Geometry check sheet. Reference: the model listing, model coordinates, mm. Face numbers are marked on the shaded views. A direction names the side the tool comes from. Give positions to 0.01 mm unless a question says otherwise; leave off trailing zeros. Write each loop counter-clockwise with the first axis right and the second up, starting at its lowest first coordinate (ties: lowest second). Pieces come first, ordered by that corner, then holes. Notation, with made-up numbers: (64, 47) -> (117, 47) arc R12 ccw to (117, 69) -> close; hole circle Ø9 at (-4.5, 5). An arc over 180 degrees is marked (long way). One line per item, written item: value.
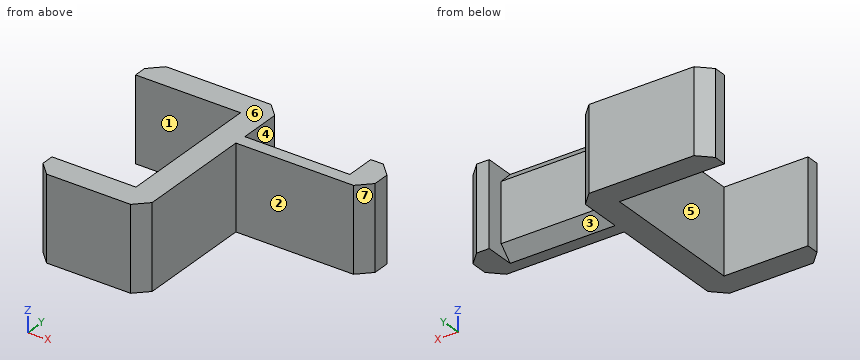
from build123d import *

# Parameters (mm, degrees)
F1_DEPTH = 20
F2_SIZE  = 3
F3_SIZE  = 3


with BuildPart() as f1:
    # F0 (on Top) → F1 (new body)
    with BuildSketch(Plane.XY):
        Polygon((-25, 6), (-25, 0), (0, 0), (0, -35), (-20, -35), (-20, -41), (6, -41), (6, -10), (37, -10), (37, 0), (31, 0), (31, -4), (6, -4), (6, 6), align=None)
    extrude(amount=F1_DEPTH)

    # F2
    f2_edges = [f1.edges().sort_by_distance(p)[0] for p in [
        (37, -10, 10),
        (6, 6, 10),
        (6, -41, 10),
        (-25, 6, 10),
        (-20, -41, 10),
        (37, 0, 10),
    ]]
    chamfer(f2_edges, length=F2_SIZE)

    # F3
    f3_edges = [f1.edges().sort_by_distance(p)[0] for p in [
        (18.5, -4, 20),
        (18.5, -4, 0),
    ]]
    chamfer(f3_edges, length=F3_SIZE)


solid = f1.part
1) Depth check by flat-ended pin: pin 1 Ø4 at (y, z) = (-13.5, 14.5) entering from -X; pin 2 Ø0.9 at (x, z) = (32.5, 8) entering from +Y; pin 3 Ø11 at (x, z) = (12.5, 8.5) entering from +Y. Enter the tip coordinate at first touch or a pass-through.
Verdict:
pin 1: x = 0
pin 2: y = 0
pin 3: y = -4
2) Sectioned sample at D-D on y = -17. Record the cut outline in (x, z), plus the area to 3 significant figures.
Verdict:
outline: (0, 0) -> (6, 0) -> (6, 20) -> (0, 20) -> close
area: 120 mm^2
3) Tool access check on the marked faces 1, 2 and 3. Record the directions out of +Z, -Z, +X, -X, +Y, -Y that give a thin tool (end or side, any length) a straight path to the whole face; none if there is none.
Verdict:
face 1: +Z, -Z, -X
face 2: +Z, -Z, +X, -Y
face 3: -Z, +Y
4) Sectioned sample at A-A on x = 7. Record the cut outline in (y, z).
Verdict:
outline: (-10, 0) -> (-7, 0) -> (-4, 3) -> (-4, 17) -> (-7, 20) -> (-10, 20) -> close
5) Sectioned sample at C-C on y = -8. Record the cut outline in (x, z), plus the area to 3 significant figures.
Verdict:
outline: (0, 0) -> (36, 0) -> (36, 20) -> (0, 20) -> close
area: 720 mm^2
6) Scan lines: probe 1 along Y at (x, z) = (-12.5, 7); probe 2 along X at (y, z) = (-11, 16); probe 3 along Y at (x, z) = (21, 17). Record each from-to range of solid material in increasing order.
Verdict:
probe 1: -41 to -35, 0 to 6
probe 2: 0 to 6
probe 3: -10 to -4
7) Sectioned sample at B-B on z = 3.75. Record the cut outline in (x, y).
Verdict:
outline: (-25, 0) -> (0, 0) -> (0, -35) -> (-20, -35) -> (-20, -38) -> (-17, -41) -> (3, -41) -> (6, -38) -> (6, -10) -> (34, -10) -> (37, -7) -> (37, -3) -> (34, 0) -> (31, 0) -> (31, -4) -> (6, -4) -> (6, 3) -> (3, 6) -> (-22, 6) -> (-25, 3) -> close
8) Mould release check, pull along X, two halves, no side actions. Record for the marked faces 4, 5, 6 and 7: released by +X, released by -X, zero draft, split by the parting line, or undercut.
Verdict:
face 4: undercut
face 5: released by -X
face 6: zero draft
face 7: released by +X
